The model under review builds one solid part; all positions refer to its coordinate system, in mm. Face numbers are marked on the shaded views. A direction names the side the tool comes from. Coordinates: 2 decimals unless noted, no trailing zeros. Order: outer loops, then holes, each group sorted by start corner. A loop starts at its lowest first (then second) coordinate and runs counter-clockwise, first axis right, second up.
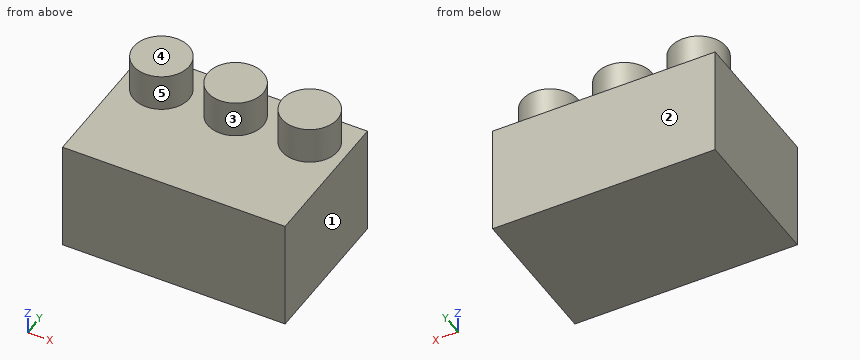
```python
from build123d import *

# Parameters (mm, degrees)
F0_W     = 76.2
F0_H     = 50.8
F1_DEPTH = 38.1
F2_R     = 9.525
F3_DEPTH = 12.7


with BuildPart() as f1:
    # F0 (on Top) → F1 (new body)
    with BuildSketch(Plane.XY):
        Rectangle(F0_W, F0_H)
    extrude(amount=F1_DEPTH)

    # F2 (on face) → F3 (join)
    with BuildSketch(Plane.XY.offset(38.1)):
        with Locations((-25.4, 12.7)):
            Circle(F2_R)
        with Locations((0, 12.7)):
            Circle(F2_R)
        with Locations((25.4, 12.7)):
            Circle(F2_R)
    extrude(amount=F3_DEPTH)


solid = f1.part
```
(1) We need section B-B, the plane x = -25.4. Write out the cut boundary in (y, z) (3 decimals).
A:
outline: (-25.4, 0) - (25.4, 0) - (25.4, 38.1) - (22.225, 38.1) - (22.225, 50.8) - (3.175, 50.8) - (3.175, 38.1) - (-25.4, 38.1) - close
(2) Machinability: for the marked faces 4 and 5, which of the approach directions +Z, -Z, +X, -X, +Y, -Y give a long, thin tool a straight path to every point of the face, cutting with its end or side? Answer none if there is none.
A:
face 4: +Z, +X, -X, +Y, -Y
face 5: +Z
(3) Wall thickness on probe 1 along X at (y, z) = (4, 44.5); probe 2 along Z at (x, y) = (-2, -14); probe 3 along X at (y, z) = (5, 40): over which ranges is each line inside the solid? List them lowest first.
A:
probe 1: x = -29.28 to -21.52, -3.88 to 3.88, 21.52 to 29.28
probe 2: z = 0 to 38.1
probe 3: x = -31.01 to -19.79, -5.61 to 5.61, 19.79 to 31.01
(4) We need section D-D, the plane y = 20. Write out the cut boundary in (x, z), and give its area (3 significant figures).
A:
outline: (-38.1, 0) - (38.1, 0) - (38.1, 38.1) - (31.52, 38.1) - (31.52, 50.8) - (19.28, 50.8) - (19.28, 38.1) - (6.12, 38.1) - (6.12, 50.8) - (-6.12, 50.8) - (-6.12, 38.1) - (-19.28, 38.1) - (-19.28, 50.8) - (-31.52, 50.8) - (-31.52, 38.1) - (-38.1, 38.1) - close
area: 3,370 mm2
(5) We need section C-C, the plane z = 41.5. Write out the cut boundary in (x, y) (3 decimals), and give its area (3 significant figures).
A:
outline: circle Ø19.05 at (-25.4, 12.7); circle Ø19.05 at (0, 12.7); circle Ø19.05 at (25.4, 12.7)
area: 855 mm2
(6) We need section A-A, the plane y = 12.7. Write out the cut boundary in (x, z) (3 decimals), and give its area (3 significant figures).
A:
outline: (-38.1, 0) - (38.1, 0) - (38.1, 38.1) - (34.925, 38.1) - (34.925, 50.8) - (15.875, 50.8) - (15.875, 38.1) - (9.525, 38.1) - (9.525, 50.8) - (-9.525, 50.8) - (-9.525, 38.1) - (-15.875, 38.1) - (-15.875, 50.8) - (-34.925, 50.8) - (-34.925, 38.1) - (-38.1, 38.1) - close
area: 3,630 mm2
(7) For pin 1 Ø4 at (x, y) = (29, -7.5) entering from +Z; pin 2 Ø1.5 at (x, z) = (4.5, 42) entering from +Y, all flat-tipped, find the tip position at first contact; note any pin that passes through.
A:
pin 1: stops at z = 38.1
pin 2: stops at y = 21.46
(8) Draft analysis for pull direction X (two halves, no side actions). For the marked faces 1, 2 and 3, state which applies: released by +X, released by -X, zero draft, split by the parting line, or undercut.
A:
face 1: released by +X
face 2: zero draft
face 3: undercut
